Source: CAD feature listing. Evaluate the final solid. Frame: model axes, mm. Face numbers are marked on the shaded views. A direction names the side the tool comes from. Round coordinates to 2 decimals unless told otherwise and drop trailing zeros. Order: outer loops, then holes, each group sorted by start corner. A loop starts at its lowest first (then second) coordinate and runs counter-clockwise, first axis right, second up.
```python
from build123d import *

# Parameters (mm, degrees)
F1_DEPTH = 3.175
F3_DEPTH = 19.05


with BuildPart() as f1:
    # F0 (on Top) → F1 (new body)
    with BuildSketch(Plane.XY):
        Polygon((-6.376508, 49.342029), (-23.076888, 49.342029), (-49.797498, 20.495921), (-47.064707, -14.423055), (-39.169982, -22.014137), (-39.169982, -33.248939), (-24.595104, -47.216527), (11.2348, -47.216527), (26.416963, -31.427078), (23.987817, 32.641653), (2.125504, 46.305597), align=None)
    extrude(amount=F1_DEPTH)

    # F2 (on face) → F3 (join)
    with BuildSketch(Plane.XY.offset(3.175)):
        Polygon((-8.460995, 27.465437), (-11.228689, 24.592964), (-11.348982, 24.524076), (-9.913685, 23.236642), (-13.435121, 19.491888), (-12.22126, 18.288707), (-13.399718, 17.099788), (-16.536398, 19.992249), (-20.168586, 19.855836), (-26.357489, 13.332929), (-26.323888, 12.755173), (-27.889514, 11.144508), (-22.5223, 5.927376), (-18.850569, 5.927376), (-17.138056, 4.265048), (-17.792482, 3.562842), (-14.112623, 0.133369), (-26.007337, -12.359691), (-19.639645, -18.486787), (-14.043322, -12.538724), (-12.448313, -14.067535), (-14.063996, -15.8737), (-11.844858, -18.042777), (-12.050118, -18.322865), (-11.044608, -19.302705), (-10.794753, -19.093755), (-9.155537, -20.661877), (-11.380946, -22.98818), (-8.972317, -25.390465), (-9.373238, -25.763512), (-6.614087, -28.535001), (-6.119217, -28.101891), (-3.923855, -30.145049), (-0.503454, -26.469847), (-0.103788, -26.803728), (4.414968, -22.089956), (3.978584, -21.701956), (6.45714, -18.914325), (3.959461, -16.693573), (4.355696, -16.247928), (1.59003, -13.500487), (1.090108, -13.844529), (-0.447387, -12.295595), (-0.811736, -12.657254), (-1.514613, -12.009452), (-1.514613, -11.054762), (-1.210493, -10.994076), (-1.318271, -9.644587), (-1.644679, -9.281886), (-1.758982, -4.754005), (-0.961826, -3.935312), (-0.075062, -4.786007), (1.278446, -3.385739), (4.118848, -3.463889), (4.094383, -2.561527), (4.542976, -2.546137), (4.551455, -2.793258), (5.533939, -2.759551), (5.525281, -2.507171), (5.788588, -2.498137), (5.778686, -2.209507), (5.589116, -2.216011), (5.582301, -2.017371), (5.014059, -2.036866), (5.014059, -1.625905), (6.536589, 0), (6.536589, 3.26362), (4.851062, 4.788233), (4.851062, 5.139193), (5.149924, 5.139193), (5.149924, 5.555849), (4.798602, 5.562526), (4.78719, 5.939749), (4.315158, 5.927964), (4.321792, 5.662222), (3.875091, 5.65107), (3.843151, 6.305763), (0.32336, 6.13405), (-0.74368, 5.033409), (-1.989887, 6.241571), (-1.989887, 7.703635), (-2.126578, 7.832781), (-2.126578, 8.485694), (-2.019443, 8.595361), (-0.881753, 8.62518), (-0.94862, 11.176316), (-2.304457, 12.350309), (-2.304457, 12.754479), (-1.808271, 12.702593), (-1.808271, 14.441202), (-2.231573, 14.441202), (-2.231573, 15.810389), (4.134082, 22.619085), (1.735728, 24.861378), (3.927975, 27.229989), (-2.817733, 33.473419), (-7.63093, 28.478006), (-8.747748, 29.554086), (-9.653301, 28.614251), align=None)
    extrude(amount=F3_DEPTH)


solid = f1.part
```
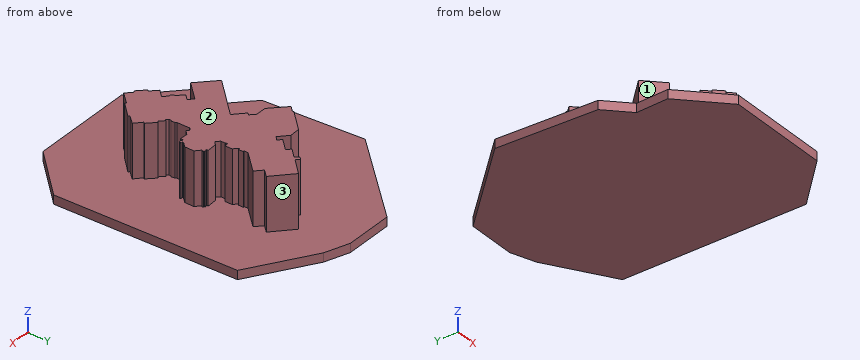
1. First-contact query: pin 1 (6 mm diameter, centred on x = -18, z = 9, fed in from -Y); pin 2 (2 mm diameter, centred on y = 11.5, z = 18.5, fed in from +X); pin 3 (8 mm diameter, centred on x = -15.5, y = 32.5, fed in from +Z) (3 decimals). Flat tips, straight axial feed; report the tip coordinate or a pass-through.
2. Line query: line 1 along Y through (x, z) = (-10, 7.5); line 2 along Y through (x, z) = (-10.5, 16.5); line 3 along Z through (x, y) = (5, -32) (3 decimals). Output: solid intervals per line, ascending.
3. Access query for the marked faces 1, 2 and 3. Directions: +Z, -Z, +X, -X, +Y, -Y. A direction counts if a zero-diameter tool reaches every point of the face in a straight line with its end or side. Return the directions, or none.
4. Section C-C on y = 37.5. Return loops of the section in (x, z) (3 decimals).
5. Section A-A on y = -6.5. Return loops of the section in (x, z) (3 decimals).
6. Section B-B on x = 21. Return loops of the section in (y, z) (3 decimals), plus the area to 3 significant figures.
Result:
1. pin 1: stops at y = -18.49
1. pin 2: stops at x = -0.93
1. pin 3: stops at z = 3.175
2. line 1: y = -24.37 to -21.54, -19.85 to 23.14, 23.31 to 25.87
2. line 2: y = -23.87 to -22.07, -19.38 to 22.61, 23.76 to 25.35
2. line 3: z = 0 to 3.175
3. face 1: +Z, -X, -Y
3. face 2: +Z, +X, -X, +Y, -Y
3. face 3: +Z, +X, +Y
4. outline: (-34.046, 0) - (16.214, 0) - (16.214, 3.175) - (-34.046, 3.175) - close
5. outline: (-47.685, 0) - (25.472, 0) - (25.472, 3.175) - (-1.715, 3.175) - (-1.715, 22.225) - (-20.428, 22.225) - (-20.428, 3.175) - (-47.685, 3.175) - close
6. outline: (-37.061, 0) - (34.509, 0) - (34.509, 3.175) - (-37.061, 3.175) - close
6. area: 227 mm2
